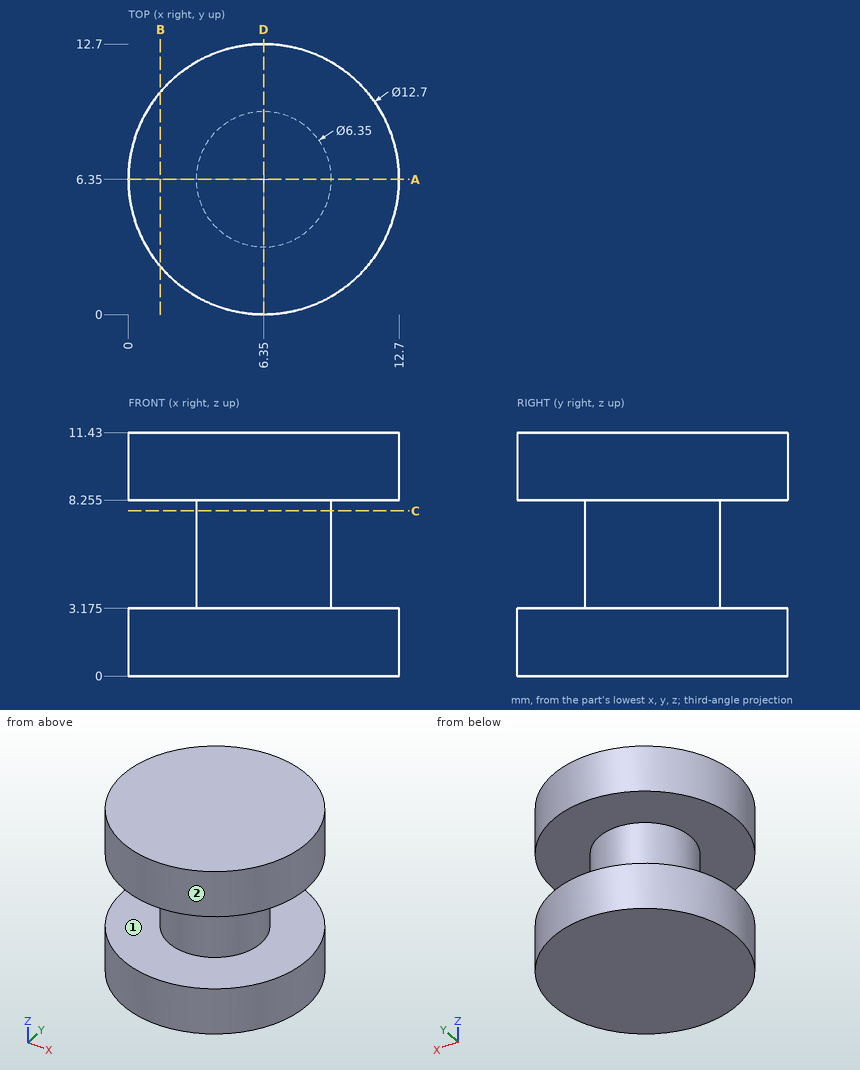
Study the drawing (mm; zero at the part's minimum x, y, z) and answer. A direction names the side the tool comes from. Give positions to 0.01 mm unless a question says otherwise; leave off trailing zeros. Write each loop counter-clockwise with the first axis right and the second up, starting at its lowest first coordinate (ties: lowest second). Pieces come first, ordered by that corner, then holes. Notation, with made-up numbers: (74.5, 61) -> (79.5, 61) arc R17 cw to (79.5, 77) -> close; hole circle Ø10 at (86, 35.25). An arc over 180 degrees is marked (long way). Answer in a Markdown table with one row per item.
1) A tool of negligible diameter and unlimited length cuts with its end or side. For the marked faces 1 and 2, from which of +Z, -Z, +X, -X, +Y, -Y can it reach the whole face along a straight path? Write none if from no direction.
Results list:
| item | result |
|---|---|
| face 1 | none |
| face 2 | +Z, -Z |
2) Section B-B on x = 1.5 is taken. Give the vertices of the cut face in (y, z) (3 decimals).
Results list:
| item | result |
|---|---|
| outline | (2.251, 0) -> (10.449, 0) -> (10.449, 3.175) -> (2.251, 3.175) -> close; (2.251, 8.255) -> (10.449, 8.255) -> (10.449, 11.43) -> (2.251, 11.43) -> close |
3) Straight lines are drawn through the part: line 1 (Z direction, x = 9.5, y = 2) (3 decimals); line 2 (X direction, y = 6.5, z = 7); line 3 (Y direction, x = 0.5, z = 2.75). For each, find the intervals that lie inside material, in ascending order. Write a range as [from, to].
Results list:
| item | result |
|---|---|
| line 1 | [0, 3.175], [8.255, 11.43] |
| line 2 | [3.18, 9.52] |
| line 3 | [3.88, 8.82] |
4) Section C-C on z = 7.75 is taken. Give the vertices of the cut face in (x, y) (3 decimals), plus the area to 3 significant figures.
Results list:
| item | result |
|---|---|
| outline | circle Ø6.35 at (6.35, 6.35) |
| area | 31.7 mm^2 |
5) Each of these flat-tipped pins is pushed along its axis until it touches: pin 1 Ø1.5 at (y, z) = (4, 7) entering from -X; pin 2 Ø1 at (y, z) = (7, 10) entering from -X; pin 3 Ø6 at (y, z) = (10, 10) entering from +X. Where does it stop, or does it pass through?
Results list:
| item | result |
|---|---|
| pin 1 | x = 3.61 |
| pin 2 | x = 0 |
| pin 3 | x = 12.67 |
6) Section A-A on y = 6.35 is taken. Give the vertices of the cut face in (x, z) (3 decimals), plus the area to 3 significant figures.
Results list:
| item | result |
|---|---|
| outline | (0, 0) -> (12.7, 0) -> (12.7, 3.175) -> (9.525, 3.175) -> (9.525, 8.255) -> (12.7, 8.255) -> (12.7, 11.43) -> (0, 11.43) -> (0, 8.255) -> (3.175, 8.255) -> (3.175, 3.175) -> (0, 3.175) -> close |
| area | 113 mm^2 |
